Source: CAD feature listing. Evaluate the final solid. Frame: model axes, mm. Face numbers are marked on the shaded views. A direction names the side the tool comes from. Give positions to 0.01 mm unless a question says otherwise; leave off trailing zeros. Order: outer loops, then holes, each group sorted by start corner. A loop starts at its lowest first (then second) coordinate and runs counter-clockwise, first axis right, second up.
1) Material intervals for line 1 (Z direction, x = 8, y = 2); line 2 (Z direction, x = 3.75, y = 2.25) (3 decimals); line 3 (Y direction, x = 3.5, z = 1.4), sorted ascending.
2) Draft query along X for the marked faces 1, 2, 3 and 4. Return one class per face: released by +X, released by -X, zero draft, split by the parting line, or undercut.
3) Section D-D, the plane x = 10. Return loops of the section in (y, z).
4) Section C-C, the plane y = 9. Return loops of the section in (x, z), plus the area to 3 significant figures.
5) Section B-B, the plane z = 35. Return loops of the section in (x, y).
6) First-contact query: P1, Ø3, axis at x = 3.5, y = 3.5, coming from the +Z side; P2, Ø1.9, axis at x = 3.5, y = 4, coming from the -Z side. Flat tips, straight axial feed; report the tip coordinate or a pass-through.
7) Section A-A, the plane y = 3.5. Return loops of the section in (x, z) (3 decimals), plus the area to 3 significant figures.
8) Access query for the marked faces 5 and 6. Directions: +Z, -Z, +X, -X, +Y, -Y. A direction counts if a zero-diameter tool reaches every point of the face in a straight line with its end or side. Return the directions, or none.
```python
from build123d import *

# Parameters (mm, degrees)
BOSS_EXTRUDE1_DEPTH     = 30
SKETCH1_13_W            = 2
SKETCH1_13_H            = 12
BOSS_EXTRUDE6_DEPTH     = 30
CUT_EXTRUDE3_DEPTH      = 5
BOSS_EXTRUDE4_START     = -2.45
BOSS_EXTRUDE4_OUTLINE_W = 30
BOSS_EXTRUDE4_OUTLINE_H = 14.485281374
BOSS_EXTRUDE4_OUTLINE_R = 1.6
BOSS_EXTRUDE4_DEPTH     = 2.45
CUT_EXTRUDE1_DEPTH      = 5
SKETCH1_10_R            = 1.7
BOSS_EXTRUDE5_DEPTH     = 2.45
CUT_EXTRUDE4_DEPTH      = 63.353829072


# Read off the part's stored shape, not the designer's step: Boss-Extrude4
with BuildPart() as part:
    # Sketch1 → Boss-Extrude1 (new body)
    with BuildSketch(Plane.XY):
        Polygon((0, 12), (12, 0), (0, 0), align=None)
    boss_extrude1 = extrude(amount=BOSS_EXTRUDE1_DEPTH)

    # Sketch1<13> → Boss-Extrude6 (add)
    with BuildSketch(Plane.XY):
        with Locations((-1, 6)):
            Rectangle(SKETCH1_13_W, SKETCH1_13_H)
    boss_extrude6 = extrude(amount=BOSS_EXTRUDE6_DEPTH)

    # Sketch4 → Cut-Extrude3 (cut)
    with BuildSketch(Plane(origin=(6, 6, 0), x_dir=(0, 0, -1), z_dir=(0.7071067811865477, 0.7071067811865475, 0))):
        Polygon((-6.175, -8.485281374), (-6.175, 3.145733136), (-9, 4.776747647), (-11.825, 3.145733136), (-11.825, -8.485281374), align=None)
    cut_extrude3 = extrude(amount=-CUT_EXTRUDE3_DEPTH, mode=Mode.SUBTRACT)

    # Boss-Extrude4 outline → Boss-Extrude4 (add)
    with BuildSketch(Plane(origin=(6, 6, 0), x_dir=(0, 0, -1), z_dir=(0.7071067811865477, 0.7071067811865475, 0)).offset(BOSS_EXTRUDE4_START)):
        with Locations((-15, -1.242640687)):
            Rectangle(BOSS_EXTRUDE4_OUTLINE_W, BOSS_EXTRUDE4_OUTLINE_H)
        with Locations((-9, 1.514718626)):
            Circle(BOSS_EXTRUDE4_OUTLINE_R, mode=Mode.SUBTRACT)
    boss_extrude4 = extrude(amount=BOSS_EXTRUDE4_DEPTH)

    # Sketch1<4> → Cut-Extrude1 (cut)
    with BuildSketch(Plane.XY):
        Polygon((10.669337222, 0), (4.440608352, 6.623473909), (1.265296423, 5.876327682), (0.324688071, 2.752853773), (2.91347758, 0), align=None)
    cut_extrude1 = extrude(amount=CUT_EXTRUDE1_DEPTH, mode=Mode.SUBTRACT)

    # Sketch1<10> → Boss-Extrude5 (add)
    # profile 1 of 2: a face of its own
    with BuildSketch(Plane.XY):
        Polygon((2.559391648, 0.376526091), (5.734703577, 1.123672318), (6.675311929, 4.247146227), (4.440608352, 6.623473909), (1.265296423, 5.876327682), (0.324688071, 2.752853773), align=None)
        with Locations((3.5, 3.5)):
            Circle(SKETCH1_10_R, mode=Mode.SUBTRACT)
    # profile 2 of 2: a face of its own
    with BuildSketch(Plane.XY):
        Polygon((3.5, 0), (10.669337222, 0), (6.675311929, 4.247146227), (5.734703577, 1.123672318), (2.559391648, 0.376526091), (2.91347758, 0), align=None)
    boss_extrude5 = extrude(amount=BOSS_EXTRUDE5_DEPTH)

    # Mirror1: Boss-Extrude1, Boss-Extrude6, Cut-Extrude3, Boss-Extrude4, Cut-Extrude1, Boss-Extrude5 across plane
    add(boss_extrude1.mirror(Plane.XY.offset(30)))
    add(boss_extrude6.mirror(Plane.XY.offset(30)))
    add(cut_extrude3.mirror(Plane.XY.offset(30)), mode=Mode.SUBTRACT)
    add(boss_extrude4.mirror(Plane.XY.offset(30)))
    add(cut_extrude1.mirror(Plane.XY.offset(30)), mode=Mode.SUBTRACT)
    add(boss_extrude5.mirror(Plane.XY.offset(30)))

    # Sketch1<12> → Cut-Extrude4 (cut, through all)
    with BuildSketch(Plane.XY):
        Polygon((12, -3.5), (12, 0), (10.669337222, 0), (3.5, 0), (2.91347758, 0), (1.441458618, 0), (0, 0), (0, -3.5), align=None)
    extrude(amount=CUT_EXTRUDE4_DEPTH, mode=Mode.SUBTRACT)


solid = part.part
```
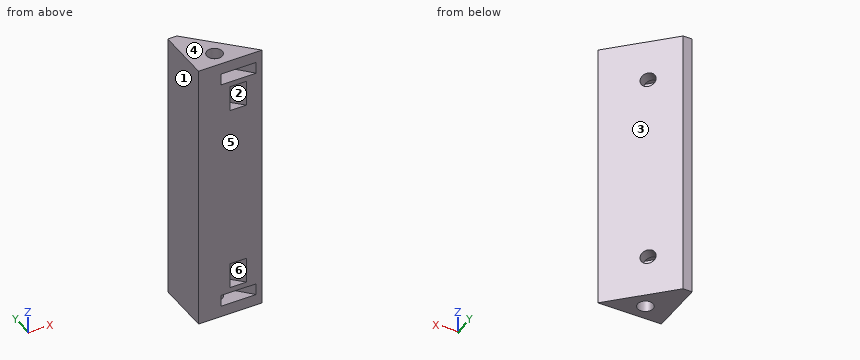
From the geometry:
1. line 1: z = 0 to 2.45, 5 to 55, 57.55 to 60
1. line 2: z = 5 to 6.175, 11.825 to 48.175, 53.825 to 55
1. line 3: y = 0 to 1.8, 5.2 to 8.5
2. face 1: released by -X
2. face 2: undercut
2. face 3: released by +X
2. face 4: zero draft
3. outline: (0, 0) - (2, 0) - (2, 60) - (0, 60) - (0, 57.55) - (0.71, 57.55) - (0.71, 55) - (0, 55) - (0, 5) - (0.71, 5) - (0.71, 2.45) - (0, 2.45) - close
4. outline: (-2, 0) - (3, 0) - (3, 60) - (-2, 60) - close
4. area: 300 mm2
5. outline: (-2, 0) - (12, 0) - (0, 12) - (-2, 12) - close
6. P1: stops at z = 55
6. P2: stops at z = 5
7. outline: (-2, 0) - (1.8, 0) - (1.8, 2.45) - (0.55, 2.45) - (0.55, 5) - (7.378, 5) - (7.378, 2.45) - (5.2, 2.45) - (5.2, 0) - (8.5, 0) - (8.5, 60) - (5.2, 60) - (5.2, 57.55) - (7.378, 57.55) - (7.378, 55) - (0.55, 55) - (0.55, 57.55) - (1.8, 57.55) - (1.8, 60) - (-2, 60) - close; hole (1.429, 6.175) - (5.035, 6.175) - (5.035, 11.825) - (1.429, 11.825) - close; hole (1.429, 48.175) - (5.035, 48.175) - (5.035, 53.825) - (1.429, 53.825) - close
7. area: 538 mm2
8. face 5: +Z, -Z, +X, -X, -Y
8. face 6: none
